Could you check a few things on this drawing? It's one solid part, dimensions in mm from its lowest x, y, z. A direction names the side the tool comes from. Coordinates: 2 decimals unless noted, no trailing zeros. Order: outer loops, then holes, each group sorted by start corner. A loop starts at its lowest first (then second) coordinate and runs counter-clockwise, first axis right, second up. Notation, with made-up numbers: (44.5, -35) -> (48.5, -35) arc R17 ccw to (48.5, -4) -> close; hole circle Ø2 at (-2.5, 30). An arc over 180 degrees is marked (long way). Use a Markdown table: item, result. Add a question column.
1. Suppose I cut it at A-A, the plane z = 18. List the corners of the cut face in (x, y) for me, then the cut area to 3 significant figures.
2. Suppose I cut it at C-C, the plane x = 5.75. State how many separate pieces and enclosed holes the cut face has, then the cut area to 3 significant figures.
3. Suppose I cut it at D-D, the plane z = 38. List the corners of the cut face in (x, y) for me.
4. For pin 1 Ø3.5 at (y, z) = (12.55, 10) entering from -X; pin 2 Ø7.5 at (y, z) = (14, 13.5) entering from -X, each with a flat end and sliding along its axis, tell me the tip position at first contact or that it passes through.
5. For the marked faces 5 and 6, which set-ups out of +Z, -Z, +X, -X, +Y, -Y let a thin tool reach every point of the face, with its end or its side?
6. If I drill on line 1 along Y through (x, z) = (6.4, 30) (1 decimal); line 2 along Z through (x, y) = (7, 12.25); line 3 along Z through (x, y) = (7.5, 12), over which ranges is the centre line in solid material (lowest first)? Write a range as from..to.
7. We'd pull the mould along Y, two halves only. Please class the marked faces 1, 2, 3 and 4: pulls with the +Y half, pulls with the -Y half, needs draft (parallel to the pull), parting line crosses it, or undercut.
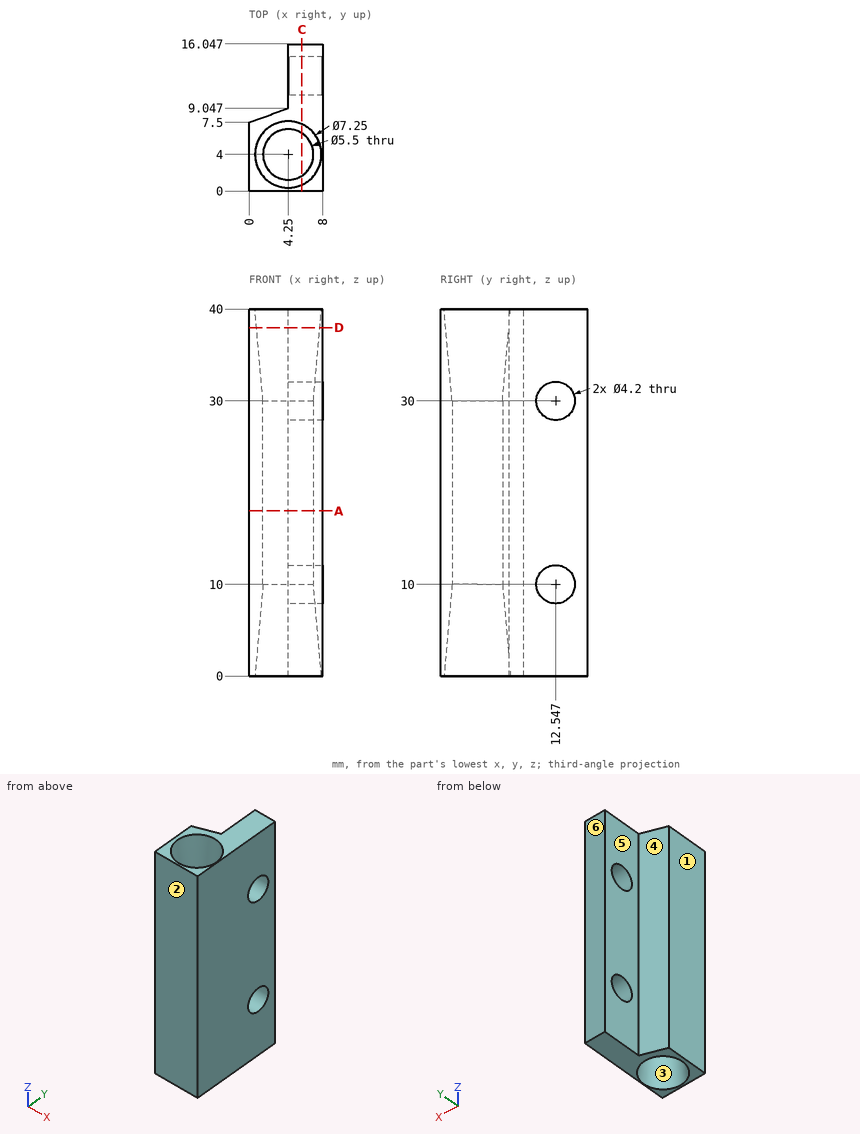
Worked out:
| question | item | result |
|---|---|---|
| 1 | outline | (0, 0) -> (8, 0) -> (8, 16.05) -> (4.25, 16.05) -> (4.25, 9.05) -> (0, 7.5) -> close; hole circle Ø5.5 at (4.25, 4) |
| 1 | area | 71.6 mm² |
| 2 | separate pieces | 2 |
| 2 | enclosed holes | 2 |
| 2 | area | 410 mm² |
| 3 | outline | (0, 0) -> (8, 0) -> (8, 16.05) -> (4.25, 16.05) -> (4.25, 9.05) -> (0, 7.5) -> close; hole circle Ø6.9 at (4.25, 4) |
| 4 | pin 1 | passes through |
| 4 | pin 2 | stops at x = 4.25 |
| 5 | face 5 | +Z, -Z, -X, +Y |
| 5 | face 6 | +Z, -Z, +X, -X, +Y |
| 6 | line 1 | y = 0..2.3, 5.7..10.4, 14.6..16 |
| 6 | line 2 | z = 0..7.92, 12.08..27.92, 32.08..40 |
| 6 | line 3 | z = 0..7.97, 12.03..27.97, 32.03..40 |
| 7 | face 1 | needs draft |
| 7 | face 2 | pulls with the -Y half |
| 7 | face 3 | undercut |
| 7 | face 4 | pulls with the +Y half |
